from build123d import *

# Parameters (mm, degrees)
SKETCH_1_W             = 224
SKETCH_1_H             = 30
EXTRUDE_1_DEPTH        = 12
SKETCH_4_R             = 5
CUT_EXTRUDE_1_DEPTH    = 227.318359839
PATTERN_LINEAR_1_COUNT = 2
PATTERN_LINEAR_1_PITCH = 137


with BuildPart() as part:
    # Sketch 1 → Бобышка-Вытянуть1 (new body)
    with BuildSketch(Plane.XY):
        with Locations((112, 15)):
            Rectangle(SKETCH_1_W, SKETCH_1_H)
    extrude(amount=EXTRUDE_1_DEPTH)

    # Эскиз4 → Вырез-Вытянуть1 (cut, symmetric)
    with BuildSketch(Plane.XY.offset(12)):
        with Locations((43.5, 15)):
            Circle(SKETCH_4_R)
    cut_extrude_1 = extrude(amount=CUT_EXTRUDE_1_DEPTH, both=True, mode=Mode.SUBTRACT)

    # Линейный массив1: Вырез-Вытянуть1 ×2
    with Locations(*[(i * PATTERN_LINEAR_1_PITCH, 0, 0) for i in range(1, PATTERN_LINEAR_1_COUNT)]):
        add(cut_extrude_1, mode=Mode.SUBTRACT)


solid = part.part
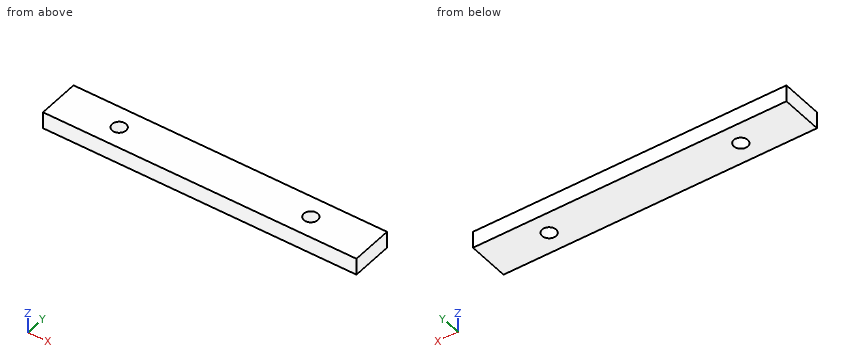
Verification items for the finished model (mm, model axes). Coordinates: 2 decimals unless noted, no trailing zeros. Loops run counter-clockwise (first coordinate to the right, second up) from the corner with the lowest first, then second, coordinate; pieces in that order, holes last. Notation, with made-up numbers: (-15, -6) -> (23, -6) arc R19 ccw to (23, 9) -> close; hole circle Ø2 at (66.5, 88.5). An arc over 180 degrees is marked (long way). Write each question's results on one line, items separated by ' | '.
Item 1: Gauge pin test, flat end, axial feed: pin 1 (8 mm diameter, centred on x = 43.5, y = 15, fed in from +Z). Record the tip position at first contact, or that the pin passes through.
Found:
pin 1: passes through
Item 2: Material ranges on L1, parallel to Y at x = 180.5, z = 4; L2, parallel to X at y = 16.25, z = 3.25; L3, parallel to X at y = 17.75, z = 8.75, recorded low to high.
Found:
L1: y = 0 to 10, 20 to 30 | L2: x = 0 to 38.66, 48.34 to 175.66, 185.34 to 224 | L3: x = 0 to 39.32, 47.68 to 176.32, 184.68 to 224
Item 3: Section check C-C, the plane z = 6.5. Enter the section's corners in (x, y), plus the area to 3 significant figures.
Found:
outline: (0, 0) -> (224, 0) -> (224, 30) -> (0, 30) -> close; hole circle Ø10 at (43.5, 15); hole circle Ø10 at (180.5, 15) | area: 6,560 mm2
Item 4: Section check B-B, the plane y = 15. Enter the section's corners in (x, z).
Found:
outline: (0, 0) -> (38.5, 0) -> (38.5, 12) -> (0, 12) -> close; (48.5, 0) -> (175.5, 0) -> (175.5, 12) -> (48.5, 12) -> close; (185.5, 0) -> (224, 0) -> (224, 12) -> (185.5, 12) -> close
Item 5: Section check A-A, the plane x = 180.5. Enter the section's corners in (y, z).
Found:
outline: (0, 0) -> (10, 0) -> (10, 12) -> (0, 12) -> close; (20, 0) -> (30, 0) -> (30, 12) -> (20, 12) -> close
